Can you work these out from the model? Positions are in its coordinate system, mm. Round coordinates to 2 decimals unless told otherwise and drop trailing zeros. Loops run counter-clockwise (first coordinate to the right, second up) from the corner with the lowest first, then second, coordinate; pieces in that order, holes last. Notation, with made-up numbers: (5, 58) -> (15, 58) arc R20 ccw to (15, 76) -> close; hole circle Ø3 at (32, 40). An arc over 180 degrees is marked (long way). Use a Markdown table: item, result.
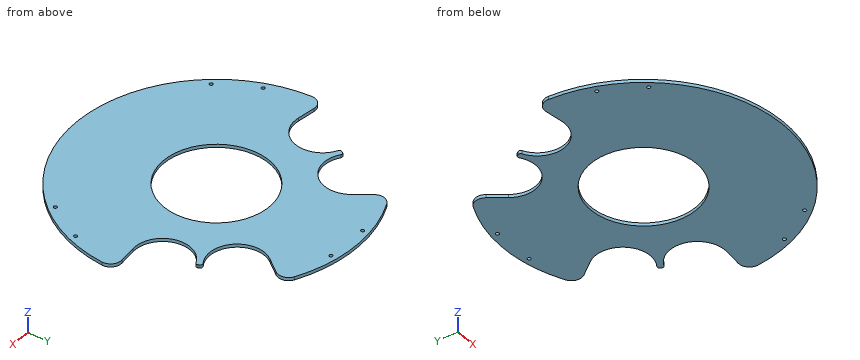
Autodesk Inventor part; units mm, degrees
ref_plane "YZ Plane" through (0, 0, 0) normal (1, 0, 0) x (0, 1, 0)
ref_plane "XZ Plane" through (0, 0, 0) normal (0, 1, 0) x (-1, 0, 0)
ref_plane "XY Plane" through (0, 0, 0) normal (0, 0, 1) x (1, 0, 0)
sketch "Эскиз1" plane through (0, 0, 0) normal (0, 0, 1) x (1, 0, 0)
  circle A0 centre (0, 0) radius 104 construction
  line L0 (0, 0) -> (0, 166.3327) construction
  line L1 (0, 0) -> (122.2993, 70.6095) construction
  line L2 (0, 0) -> (95.803, 99.2069) construction
  line L3 (0, 0) -> (133.5999, 33.3102) construction
  circle A1 centre (72.2445, 74.8113) radius 26
  circle A2 centre (100.9108, 25.1599) radius 26
  circle A3 centre (0, 0) radius 132.5
  line L4 (51.4307, 90.3929) -> (68.6163, 113.3493)
  line L5 (88.543, 54.554) -> (110.8856, 72.5303)
  line L6 (91.5167, 49.4035) -> (118.2559, 59.7646)
  line L7 (103.9979, -0.6562) -> (132.4715, 2.7488)
  circle A4 centre (-72.2445, 74.8113) radius 26
  circle A5 centre (-100.9108, 25.1599) radius 26
  line L8 (-51.4307, 90.3929) -> (-68.6163, 113.3493)
  line L9 (-88.543, 54.554) -> (-110.8856, 72.5303)
  line L10 (-91.5167, 49.4035) -> (-118.2559, 59.7646)
  line L11 (-103.9979, -0.6562) -> (-132.4715, 2.7488)
  arc A6 (91.5167, 49.4035) -> (88.543, 54.554) centre (0, 0) ccw
  arc A7 (-88.543, 54.554) -> (-91.5167, 49.4035) centre (0, 0) ccw
  point P0 (-68.6163, 113.3493)
  point P1 (-110.8856, 72.5303)
  point P2 (-118.2559, 59.7646)
  point P3 (-132.4715, 2.7488)
  dimension "d0" = 208
  dimension "d1" = 52
  dimension "d2" = 32
  dimension "d3" = 60
  dimension "d4" = 265
extrude "Выдавливание1" add sketch "Эскиз1" along normal mid plane 3 contours A1 A6 A2 L7 A3 L11 A5 A7 A4 L8 L4
fillet "Сопряжение1" radius 10 4 edges at (-68.6163, 113.3493, 0) (-132.4715, 2.7488, 0) (68.6163, 113.3493, 0) (132.4715, 2.7488, 0)
fillet "Сопряжение1" radius 2 4 edges at (88.543, 54.554, 0) (91.5167, 49.4035, 0) (-88.543, 54.554, 0) (-91.5167, 49.4035, 0)
sketch "Эскиз2" plane through (0, 0, 1.5) normal (0, 0, 1) x (1, 0, 0)
  circle A0 centre (20, 124.909) radius 1.95 construction
  circle A1 centre (20, 124.909) radius 1.6
  circle A2 centre (-20, 124.909) radius 1.6
  circle A3 centre (-20, 124.909) radius 1.6
  point P0 (0, 0)
  dimension "d9" = 3.2
extrude "Выдавливание2" cut sketch "Эскиз2" against normal through all
pattern_circular "Круговой массив1" count 3 over 360 about axis through (0, 0, -10) along (0, 0, 1) of "Выдавливание2"
sketch "Эскиз3" plane through (0, 0, 1.5) normal (0, 0, 1) x (1, 0, 0)
  circle A0 centre (0, 0) radius 50
  dimension "d15" = 100
extrude "Выдавливание3" cut sketch "Эскиз3" against normal through all
properties part number "Диск_фиксирующий"
1. I want a section at A-A (x = 0). Please give me the cut outline in (y, z).
Answer sheet:
| item | result |
|---|---|
| outline | (-132.5, -1.5) -> (-50, -1.5) -> (-50, 1.5) -> (-132.5, 1.5) -> close; (50, -1.5) -> (132.5, -1.5) -> (132.5, 1.5) -> (50, 1.5) -> close |
2. I want a section at C-C (y = 84). Please give me the cut outline in (x, z).
Answer sheet:
| item | result |
|---|---|
| outline | (-47.92, -1.5) -> (47.92, -1.5) -> (47.92, 1.5) -> (-47.92, 1.5) -> close |
3. I want a section at D-D (z = 0.25). State how many separate pieces and enclosed holes the cut face has, plus the area to 3 significant figures.
Answer sheet:
| item | result |
|---|---|
| separate pieces | 1 |
| enclosed holes | 7 |
| area | 36,200 mm² |
4. Will these pins go through, and if not, where does the flat tip stop? pin 1 Ø1.5 at (y, z) = (-82, 0.5) entering from +X; pin 2 Ø1 at (y, z) = (-97.5, 0.5) entering from +X; pin 3 Ø1 at (y, z) = (55.5, -0.5) entering from +X.
Answer sheet:
| item | result |
|---|---|
| pin 1 | stops at x = 104.66 |
| pin 2 | stops at x = 90.26 |
| pin 3 | stops at x = 55.41 |
5. I need wall thicknesses on line 1 (Y direction, x = 0, z = 0.8); line 2 (X direction, y = 51, z = -1.1); line 3 (X direction, y = -6, z = -1.25). Which ranges of each line are inside material? Lowest first, please.
Answer sheet:
| item | result |
|---|---|
| line 1 | y = -132.5 to -50, 50 to 132.5 |
| line 2 | x = -90.6 to -82.69, -61.8 to 61.8, 82.69 to 90.6 |
| line 3 | x = -131.87 to -49.64, 49.64 to 131.87 |
6. I want a section at B-B (x = 81). Please give me the cut outline in (y, z), plus the area to 3 significant figures.
Answer sheet:
| item | result |
|---|---|
| outline | (-104.86, -1.5) -> (8.44, -1.5) -> (8.44, 1.5) -> (-104.86, 1.5) -> close; (41.88, -1.5) -> (50.33, -1.5) -> (50.33, 1.5) -> (41.88, 1.5) -> close |
| area | 365 mm² |
